Geometry: see drawing. Coordinates: mm, zero at the bounding-box minimum. A direction names the side the tool comes from. Give positions to 0.01 mm unless a question says otherwise; leave off trailing zeros. Write each loop counter-clockwise with the first axis right and the second up, starting at its lowest first coordinate (ties: lowest second). Pieces come first, ordered by that corner, then holes. Notation, with made-up numbers: (42.5, -18) - (81.5, -18) arc R14 ccw to (81.5, 6) - close; hole circle Ø8 at (-15, 46.5). An arc over 180 degrees is marked (long way). Return JSON: item names as keys, results as strings.
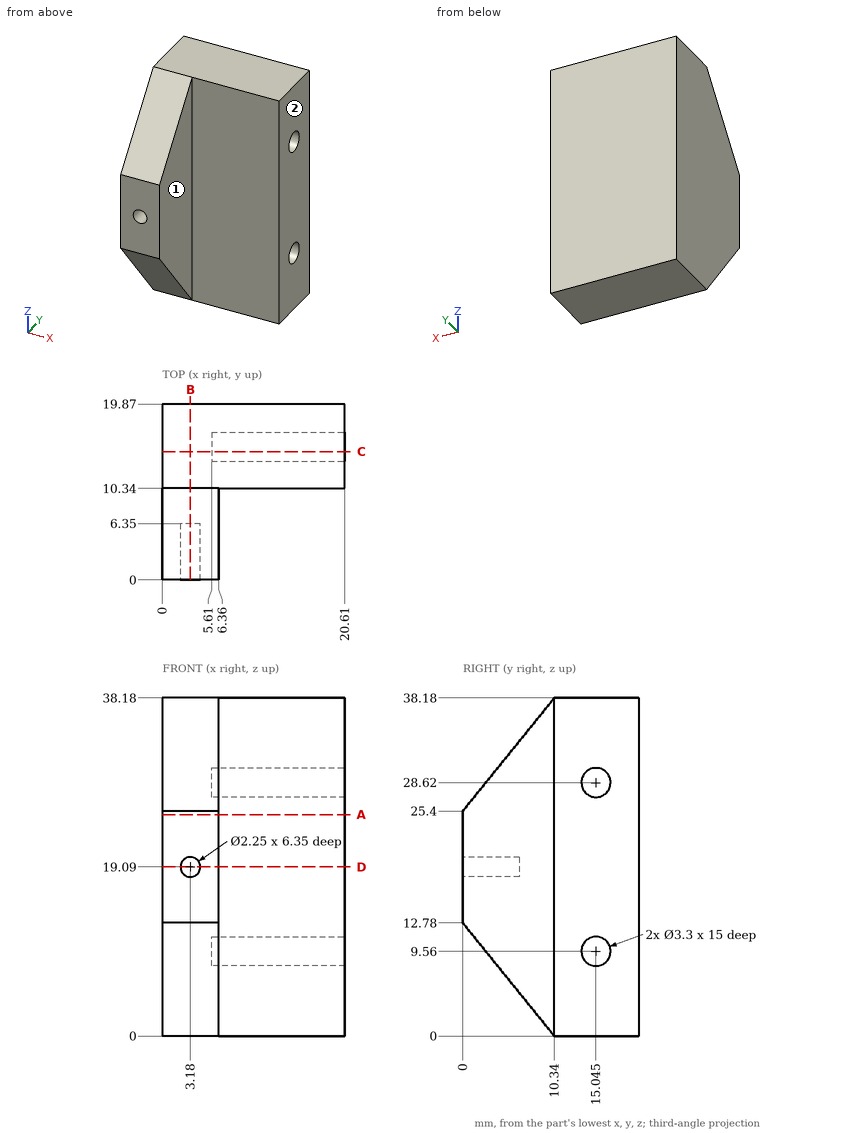
Q1. Section query D-D, the plane z = 19.09. Return the cut outline in (x, y) (3 decimals), plus the area to 3 significant figures.
Answer key:
{"outline": "(0, 0) - (2.055, 0) - (2.055, 6.35) - (4.305, 6.35) - (4.305, 0) - (6.36, 0) - (6.36, 10.34) - (20.61, 10.34) - (20.61, 19.87) - (0, 19.87) - close", "area": "248 mm^2"}
Q2. Set-up query: the marked faces 1 and 2. Return all of +Z, -Z, +X, -X, +Y, -Y with unobstructed straight access to the full face (end or side cutting, diameter ignored); none if empty.
Answer key:
{"face 1": "+Z, -Z, +X, -Y", "face 2": "+Z, -Z, +X, +Y, -Y"}
Q3. Section query C-C, the plane y = 14.5. Return the cut outline in (x, z).
Answer key:
{"outline": "(0, 0) - (20.61, 0) - (20.61, 8) - (5.61, 8) - (5.61, 11.12) - (20.61, 11.12) - (20.61, 27.06) - (5.61, 27.06) - (5.61, 30.18) - (20.61, 30.18) - (20.61, 38.18) - (0, 38.18) - close"}
Q4. Pin query (flat end, axial travel): P1, Ø1.1, axis at x = 3.5, z = 19.5, coming from the -Y side; P2, Ø4.5, axis at x = 14, z = 25.5, coming from the -Y side; P3, Ø1.6, axis at y = 15, z = 9, coming from the +X side. Return the tip coordinate at first contact, or that it passes through.
Answer key:
{"P1": "stops at y = 6.35", "P2": "stops at y = 10.34", "P3": "stops at x = 5.61"}
Q5. Material intervals for probe 1 along Z at (x, y) = (14.5, 15); probe 2 along X at (y, z) = (7.5, 14); probe 3 along Z at (x, y) = (3.18, 5) (3 decimals), sorted ascending. Write a range as [from, to].
Answer key:
{"probe 1": "z = [0, 7.91], [11.21, 26.97], [30.27, 38.18]", "probe 2": "x = [0, 6.36]", "probe 3": "z = [6.6, 17.965], [20.215, 31.58]"}
Q6. Section query A-A, the plane z = 25. Return the cut outline in (x, y), plus the area to 3 significant figures.
Answer key:
{"outline": "(0, 0) - (6.36, 0) - (6.36, 10.34) - (20.61, 10.34) - (20.61, 19.87) - (0, 19.87) - close", "area": "262 mm^2"}
Q7. Section query B-B, the plane x = 3.18. Return the cut outline in (y, z) (3 decimals), plus the area to 3 significant figures.
Answer key:
{"outline": "(0, 12.78) - (10.34, 0) - (19.87, 0) - (19.87, 38.18) - (10.34, 38.18) - (0, 25.4) - (0, 20.215) - (6.35, 20.215) - (6.35, 17.965) - (0, 17.965) - close", "area": "612 mm^2"}
